Can you work these out from the model? Positions are in its coordinate system, mm. A direction names the side the tool comes from. Give positions to 0.01 mm unless a question says otherwise; leave off trailing zeros. Loops run counter-clockwise (first coordinate to the right, second up) from the corner with the lowest first, then second, coordinate; pieces in that order, holes last. Notation, with made-up numbers: (56.5, -22) - (85.5, -22) arc R19 cw to (85.5, 12) - close; hole circle Ø2 at (72.5, -20.75). An arc over 180 degrees is marked (long way). Answer as a JSON object with one key per item and string values. Group by question number.
Item 1: Suppose I cut it at A-A on y = 0. Write out the boundary of the cut face in (x, z) (3 decimals), and give its area (3 significant figures).
Item 2: Suppose I cut it at B-B on x = 8. Write out the boundary of the cut face in (y, z) (3 decimals), and give its area (4 significant figures).
Item 3: Thinking about a two-plate mould opening in X: for faces 4 (the flat face through (-11, 0, 0)), 5 (the flat face through (-10.15, 0, 5)), 6 (the cylindrical face through (25.245, 17.796, 5.063)), which applies, pulls with the +X half, pulls with the -X half, needs draft (parallel to the pull), parting line crosses it, or undercut?
Item 4: Which directions (+Z, -Z, +X, -X, +Y, -Y) give clear straight access to the entire face, cutting with the end or side of a thin tool? Please do faces 1 (the flat face through (0, -10.15, 5)), 2 (the flat face through (17.35, 0, 2)), 3 (the cylindrical face through (21.875, -21.965, 4.937)).
Item 5: Please list where these lines run through material, in increasing order: L1, parallel to Y at x = 15.25, z = 5 (3 decimals); L2, parallel to Y at x = 6, z = 7.75 (3 decimals).
Item 6: Will this pin go through, and if not, where does the flat tip stop? pin 1 (3.5 mm diameter, centred on y = 0, z = 5, fed in from +X).
from build123d import *

# Parameters (mm, degrees)
SKIZZE1_W                       = 20.3
SKIZZE1_H                       = 20.3
AUFSATZ_LINEAR_AUSTRAGEN1_DEPTH = 10
VERRUNDUNG1_R                   = 0.2
VERRUNDUNG2_R                   = 2.5
SCHNITT_LINEAR_AUSTRAGEN1_REACH = 52.75
SKIZZE2_R                       = 2.3
CUT_EXTRUDE2_START              = -50.75
SKETCH1_2_R                     = 3.75
CUT_EXTRUDE2_DEPTH              = 8.025
FASE2_SIZE                      = 0.5


with BuildPart() as part:
    # Skizze1 → Aufsatz-Linear austragen1 (new body)
    with BuildSketch(Plane.XY):
        with BuildLine():
            Line((17.807565106, 25.375), (-17.807565106, 25.375))
            ThreePointArc((-17.807565106, 25.375), (-21.920310217, 21.920310217), (-25.375, 17.807565106))
            Line((-25.375, 17.807565106), (-25.375, -17.807565106))
            ThreePointArc((-25.375, -17.807565106), (-21.920310217, -21.920310217), (-17.807565106, -25.375))
            Line((-17.807565106, -25.375), (17.807565106, -25.375))
            ThreePointArc((17.807565106, -25.375), (21.920310217, -21.920310217), (25.375, -17.807565106))
            Line((25.375, -17.807565106), (25.375, 17.807565106))
            ThreePointArc((25.375, 17.807565106), (21.920310217, 21.920310217), (17.807565106, 25.375))
        make_face()
        Rectangle(SKIZZE1_W, SKIZZE1_H, mode=Mode.SUBTRACT)
    extrude(amount=AUFSATZ_LINEAR_AUSTRAGEN1_DEPTH)

    # Verrundung1
    verrundung1_edges = [part.edges().sort_by_distance(p)[0] for p in [
        (10.15, -10.15, 5),
        (10.15, 10.15, 5),
        (-10.15, 10.15, 5),
        (-10.15, -10.15, 5),
    ]]
    fillet(verrundung1_edges, radius=VERRUNDUNG1_R)

    # Verrundung2
    verrundung2_edges = [part.edges().sort_by_distance(p)[0] for p in [
        (25.375, 17.807565106, 5),
        (25.375, -17.807565106, 5),
        (17.807565106, -25.375, 5),
        (-17.807565106, -25.375, 5),
        (-25.375, -17.807565106, 5),
        (-25.375, 17.807565106, 5),
        (-17.807565106, 25.375, 5),
        (17.807565106, 25.375, 5),
    ]]
    fillet(verrundung2_edges, radius=VERRUNDUNG2_R)

    # Skizze2 → Schnitt-Linear austragen1 (cut, up to next)
    with BuildSketch(Plane(origin=(25.375, 0, 0), x_dir=(0, 0, -1), z_dir=(1, 0, 0)), mode=Mode.PRIVATE) as schnitt_linear_austragen1_sk1:
        with Locations((-5, 0)):
            Circle(SKIZZE2_R)
    schnitt_linear_austragen1_tool1 = extrude(schnitt_linear_austragen1_sk1.sketch, amount=-SCHNITT_LINEAR_AUSTRAGEN1_REACH, mode=Mode.PRIVATE) & part.part
    add(schnitt_linear_austragen1_tool1.solids().sort_by_distance((25.375, 0, 5))[0], mode=Mode.SUBTRACT)

    # Sketch1<2> → Cut-Extrude2 (cut)
    with BuildSketch(Plane.ZY.offset(25.375).offset(CUT_EXTRUDE2_START)):
        with Locations((5, 0)):
            Circle(SKETCH1_2_R)
    extrude(amount=CUT_EXTRUDE2_DEPTH, mode=Mode.SUBTRACT)

    # Fase2
    fase2_edges = [part.edges().sort_by_distance(p)[0] for p in [
        (10.15, 0, 7.3),
        (17.35, 0, 7.3),
        (0, -10.15, 0),
        (0, -10.15, 10),
        (10.15, 0, 0),
        (10.15, 0, 10),
        (-10.15, 0, 0),
        (-10.15, 0, 10),
        (0, 10.15, 0),
        (0, 10.15, 10),
        (10.091421356, -10.091421356, 0),
        (10.091421356, -10.091421356, 10),
        (-10.091421356, -10.091421356, 0),
        (-10.091421356, -10.091421356, 10),
        (-10.091421356, 10.091421356, 0),
        (-10.091421356, 10.091421356, 10),
        (10.091421356, 10.091421356, 0),
        (10.091421356, 10.091421356, 10),
        (0, 25.375, 0),
        (0, 25.375, 10),
        (21.920310217, 21.920310217, 0),
        (25.375, 0, 0),
        (21.920310217, -21.920310217, 0),
        (0, -25.375, 0),
        (-21.920310217, -21.920310217, 0),
        (-25.375, 0, 0),
        (-21.920310217, 21.920310217, 0),
        (-17.784891513, 25.248441317, 0),
        (-25.248441317, 17.784891513, 0),
        (-25.248441317, -17.784891513, 0),
        (-17.784891513, -25.248441317, 0),
        (17.784891513, -25.248441317, 0),
        (25.248441317, -17.784891513, 0),
        (25.248441317, 17.784891513, 0),
        (17.784891513, 25.248441317, 0),
        (21.920310217, 21.920310217, 10),
        (-21.920310217, 21.920310217, 10),
        (-25.375, 0, 10),
        (-21.920310217, -21.920310217, 10),
        (0, -25.375, 10),
        (21.920310217, -21.920310217, 10),
        (25.375, 0, 10),
        (-17.784891513, 25.248441317, 10),
        (-25.248441317, 17.784891513, 10),
        (-25.248441317, -17.784891513, 10),
        (-17.784891513, -25.248441317, 10),
        (17.784891513, -25.248441317, 10),
        (25.248441317, -17.784891513, 10),
        (25.248441317, 17.784891513, 10),
        (17.784891513, 25.248441317, 10),
    ]]
    chamfer(fase2_edges, length=FASE2_SIZE)


solid = part.part
Worked out:
{
 "1": {"outline": "(-25.375, 0.5) - (-24.875, 0) - (-10.65, 0) - (-10.15, 0.5) - (-10.15, 9.5) - (-10.65, 10) - (-24.875, 10) - (-25.375, 9.5) - close; (10.15, 0.5) - (10.65, 0) - (24.875, 0) - (25.375, 0.5) - (25.375, 1.25) - (17.35, 1.25) - (17.35, 2.2) - (16.85, 2.7) - (10.65, 2.7) - (10.15, 2.2) - close; (10.15, 7.8) - (10.65, 7.3) - (16.85, 7.3) - (17.35, 7.8) - (17.35, 8.75) - (25.375, 8.75) - (25.375, 9.5) - (24.875, 10) - (10.65, 10) - (10.15, 9.5) - close", "area": "210 mm2"},
 "2": {"outline": "(-25.375, 0.5) - (-24.875, 0) - (-10.65, 0) - (-10.15, 0.5) - (-10.15, 9.5) - (-10.65, 10) - (-24.875, 10) - (-25.375, 9.5) - close; (10.15, 0.5) - (10.65, 0) - (24.875, 0) - (25.375, 0.5) - (25.375, 9.5) - (24.875, 10) - (10.65, 10) - (10.15, 9.5) - close", "area": "303.5 mm2"},
 "3": {"face 4": "needs draft", "face 5": "undercut", "face 6": "pulls with the +X half"},
 "4": {"face 1": "+Z, -Z", "face 2": "+X", "face 3": "+Z, -Z, +X, -Y"},
 "5": {"L1": "y = -25.375 to -2.3, 2.3 to 25.375", "L2": "y = -25.375 to -10.15, 10.15 to 25.375"},
 "6": {"pin 1": "stops at x = -10.15"}
}
